Model file for the job. Use its own axes, mm. Give positions to 0.01 mm unless a question says otherwise; leave off trailing zeros. Write each loop counter-clockwise with the first axis right and the second up, starting at its lowest first coordinate (ties: lowest second). Pieces come first, ordered by that corner, then holes. Notation, with made-up numbers: (10.5, 69.5) - (29.5, 69.5) arc R18 ccw to (29.5, 75.5) - close; hole circle Ø10 at (0.25, 43). An arc over 180 degrees is marked (long way). Use CSV: the item, a comma, the result in double quotes.
from build123d import *

# Parameters (mm, degrees)
SKETCH1_W           = 34.925
SKETCH1_H           = 73.025
BOSS_EXTRUDE1_DEPTH = 1.5875
SKETCH1_4_R         = 1.4732
CUT_EXTRUDE1_DEPTH  = 1.5875


with BuildPart() as part:
    # Sketch1 → Boss-Extrude1 (new body)
    with BuildSketch(Plane(origin=(0, 0, 0), x_dir=(1, 0, 0), z_dir=(0, 1, 0))):
        with Locations((17.4625, 36.5125)):
            Rectangle(SKETCH1_W, SKETCH1_H)
    extrude(amount=BOSS_EXTRUDE1_DEPTH)

    # Sketch1_4 → Cut-Extrude1 (cut)
    with BuildSketch(Plane(origin=(0, 0, 0), x_dir=(1, 0, 0), z_dir=(0, 1, 0))):
        with Locations(Location((31.75, 69.85, 0), (0, 0, 270))):
            Circle(SKETCH1_4_R)
        with Locations(Location((3.175, 69.85, 0), (0, 0, 270))):
            Circle(SKETCH1_4_R)
        with Locations(Location((31.75, 3.175, 0), (0, 0, 270))):
            Circle(SKETCH1_4_R)
        with Locations(Location((3.175, 3.175, 0), (0, 0, 270))):
            Circle(SKETCH1_4_R)
    extrude(amount=CUT_EXTRUDE1_DEPTH, mode=Mode.SUBTRACT)


solid = part.part
(1) Flat gauge pins, fed straight in: P1, Ø3.5, axis at x = 31.75, z = -69.85, coming from the +Y side; P2, Ø1.8, axis at x = 3.175, z = -3.175, coming from the -Y side. Where does each tip first touch, or does it go through?
Checked values:
P1,"stops at y = 1.59"
P2,"passes through"
(2) Saw through at A-A, the plane z = -69.85. List the corners of the cut face in (x, y) (1 decimal).
Checked values:
outline,"(0, 0) - (1.7, 0) - (1.7, 1.6) - (0, 1.6) - close; (4.6, 0) - (30.3, 0) - (30.3, 1.6) - (4.6, 1.6) - close; (33.2, 0) - (34.9, 0) - (34.9, 1.6) - (33.2, 1.6) - close"
(3) Pull direction X, two halves, no side cores. Call faces 1 (the face through (17, 1, 0)), 2 (the face through (34.925, 1, -36)), 3 (the face through (2.279, 0.783, -4.344)), 4 (the face through (30.31, 0.78, -3.49)): released by +X, released by -X, zero draft, split by the parting line, or undercut.
Checked values:
face 1,"zero draft"
face 2,"released by +X"
face 3,"undercut"
face 4,"undercut"
(4) Wall check: probe 1 along X at (y, z) = (0.95, -69.85) (3 decimals); probe 2 along Z at (x, y) = (2, 1.55) (3 decimals); probe 3 along X at (y, z) = (0.45, -4.5) (3 decimals). Give the ranges that are in metal, low to high. Write a range as [from, to].
Checked values:
probe 1,"x = [0, 1.702], [4.648, 30.277], [33.223, 34.925]"
probe 2,"z = [-73.025, -70.739], [-68.961, -4.064], [-2.286, 0]"
probe 3,"x = [0, 2.531], [3.819, 31.106], [32.394, 34.925]"
(5) Saw through at B-B, the plane x = 31.75. List the corners of the cut face in (y, z) (1 decimal), then the cut area to 3 significant figures.
Checked values:
outline,"(0, -73) - (1.6, -73) - (1.6, -71.3) - (0, -71.3) - close; (0, -68.4) - (1.6, -68.4) - (1.6, -4.6) - (0, -4.6) - close; (0, -1.7) - (1.6, -1.7) - (1.6, 0) - (0, 0) - close"
area,"107 mm^2"
